from build123d import *

# Parameters (mm, degrees)
SKETCH_1_W      = 120
SKETCH_1_H      = 20
SKETCH_1_R      = 2.5
EXTRUDE_1_DEPTH = 4


with BuildPart() as part:
    # Эскиз1 → Бобышка-Вытянуть1 (new body)
    with BuildSketch(Plane(origin=(0, 0, 0), x_dir=(0, 0, -1), z_dir=(1, 0, 0))):
        with Locations((60, 10)):
            Rectangle(SKETCH_1_W, SKETCH_1_H)
        with Locations((110, 15)):
            Circle(SKETCH_1_R, mode=Mode.SUBTRACT)
        with Locations((110, 5)):
            Circle(SKETCH_1_R, mode=Mode.SUBTRACT)
        with Locations((14, 15)):
            Circle(SKETCH_1_R, mode=Mode.SUBTRACT)
        with Locations((14, 5)):
            Circle(SKETCH_1_R, mode=Mode.SUBTRACT)
    extrude(amount=EXTRUDE_1_DEPTH)


solid = part.part
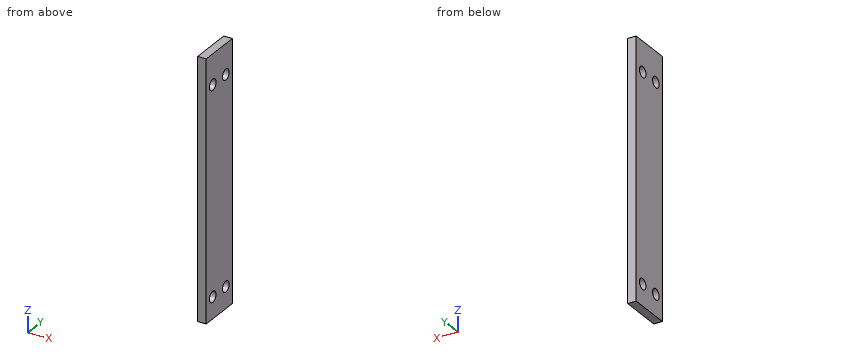
Can you work these out from the model? Positions are in its coordinate system, mm. Round coordinates to 2 decimals unless told otherwise and drop trailing zeros. Loops run counter-clockwise (first coordinate to the right, second up) from the corner with the lowest first, then second, coordinate; pieces in that order, holes last. Notation, with made-up numbers: (51.25, 30.5) - (60.25, 30.5) arc R4 cw to (60.25, 37.5) - close; hole circle Ø6 at (89, 40). An arc over 180 degrees is marked (long way). Answer in a Markdown table with one row per item. Add a question column.
Q1. I want a section at B-B on x = 2.25. List the corners of the cut face in (y, z) for me, and give its area (3 significant figures).
Q2. I need wall thicknesses on L1, parallel to Y at x = 1.25, z = -110; L2, parallel to Z at x = 3.2, y = 16.25; L3, parallel to Z at x = 0.65, y = 17.25. Which ranges of each line are inside material? Lowest first, please.
Q3. I want a section at A-A on z = -110. List the corners of the cut face in (x, y) for me, and give its area (3 significant figures).
Q4. I want a section at C-C on y = 15. List the corners of the cut face in (x, z) for me, and give its area (3 significant figures).
A:
| question | item | result |
|---|---|---|
| 1 | outline | (0, -120) - (20, -120) - (20, 0) - (0, 0) - close; hole circle Ø5 at (5, -110); hole circle Ø5 at (5, -14); hole circle Ø5 at (15, -110); hole circle Ø5 at (15, -14) |
| 1 | area | 2,320 mm^2 |
| 2 | L1 | 0 to 2.5, 7.5 to 12.5, 17.5 to 20 |
| 2 | L2 | -120 to -112.17, -107.83 to -16.17, -11.83 to 0 |
| 2 | L3 | -120 to -111.09, -108.91 to -15.09, -12.91 to 0 |
| 3 | outline | (0, 0) - (4, 0) - (4, 2.5) - (0, 2.5) - close; (0, 7.5) - (4, 7.5) - (4, 12.5) - (0, 12.5) - close; (0, 17.5) - (4, 17.5) - (4, 20) - (0, 20) - close |
| 3 | area | 40.0 mm^2 |
| 4 | outline | (0, -120) - (4, -120) - (4, -112.5) - (0, -112.5) - close; (0, -107.5) - (4, -107.5) - (4, -16.5) - (0, -16.5) - close; (0, -11.5) - (4, -11.5) - (4, 0) - (0, 0) - close |
| 4 | area | 440 mm^2 |
